The model under review builds one solid part; all positions refer to its coordinate system, in mm. Coordinates: 2 decimals unless noted, no trailing zeros. Write each loop counter-clockwise with the first axis right and the second up, starting at its lowest first coordinate (ties: lowest second). Pieces come first, ordered by that corner, then holes. Notation, with made-up numbers: (41, -37) - (88, -37) arc R10 cw to (88, -26) - close; hole circle Ø6 at (56, 26.25). An arc over 180 degrees is marked (long way). Put each result on its own line as item: value. Start each with the question number.
Item 1: Consider section B-B on y = 0.3. Give the boundary of the cut face in (x, z), then the cut area to 3 significant figures.
Item 2: Consider section A-A on z = 0. Give the boundary of the cut face in (x, y).
Item 3: To check wall thickness, follow L1, parallel to X at y = 1, z = 0; L2, parallel to Z at x = -6.25, y = 0.45; L3, parallel to X at y = 0.4, z = 4.5. State the ranges of each line that lie inside material, in increasing order. Write a range as [from, to].
Item 4: Consider section D-D on x = 0. Give the boundary of the cut face in (y, z), then the cut area to 3 significant figures.
Item 5: Consider section C-C on z = 3. Give the boundary of the cut face in (x, y), then the cut area to 3 significant figures.
```python
from build123d import *

# Parameters (mm, degrees)
EXTRUDE1_DEPTH = 1.2


with BuildPart() as part:
    # Sketch1 → Extrude1 (new body)
    with BuildSketch(Plane(origin=(0, 0, 0), x_dir=(1, 0, 0), z_dir=(0, 1, 0))):
        with BuildLine():
            Line((2.113091309, 4.531538935), (2.371939111, 5.086639839))
            ThreePointArc((2.371939111, 5.086639839), (3.208308367, 5.77268928), (4.266742072, 5.549316362))
            ThreePointArc((4.266742072, 5.549316362), (5.73406431, 4.015035054), (6.673963371, 2.111448062))
            ThreePointArc((6.673963371, 2.111448062), (6.515398476, 1.030863961), (5.568082875, 0.487358691))
            Line((5.568082875, 0.487358691), (4.979992479, 0.446849981))
            ThreePointArc((4.979992479, 0.446849981), (4.742221478, -1.58471936), (3.710828514, -3.351082175))
            Line((3.710828514, -3.351082175), (4.262184676, -6.810891939))
            ThreePointArc((4.262184676, -6.810891939), (5.05662557, -7.784180304), (6.29553407, -7.575536336))
            ThreePointArc((6.29553407, -7.575536336), (0, 9.85), (-6.29553407, -7.575536336))
            ThreePointArc((-6.29553407, -7.575536336), (-5.05662557, -7.784180304), (-4.262184676, -6.810891939))
            Line((-4.262184676, -6.810891939), (-3.710828514, -3.351082175))
            ThreePointArc((-3.710828514, -3.351082175), (-4.742221478, -1.58471936), (-4.979992479, 0.446849981))
            Line((-4.979992479, 0.446849981), (-5.568082875, 0.487358691))
            ThreePointArc((-5.568082875, 0.487358691), (-6.515398476, 1.030863961), (-6.673963371, 2.111448062))
            ThreePointArc((-6.673963371, 2.111448062), (-5.73406431, 4.015035054), (-4.266742072, 5.549316362))
            ThreePointArc((-4.266742072, 5.549316362), (-3.208308367, 5.77268928), (-2.371939111, 5.086639839))
            Line((-2.371939111, 5.086639839), (-2.113091309, 4.531538935))
            ThreePointArc((-2.113091309, 4.531538935), (0, 5), (2.113091309, 4.531538935))
        make_face()
    extrude(amount=EXTRUDE1_DEPTH)


solid = part.part
```
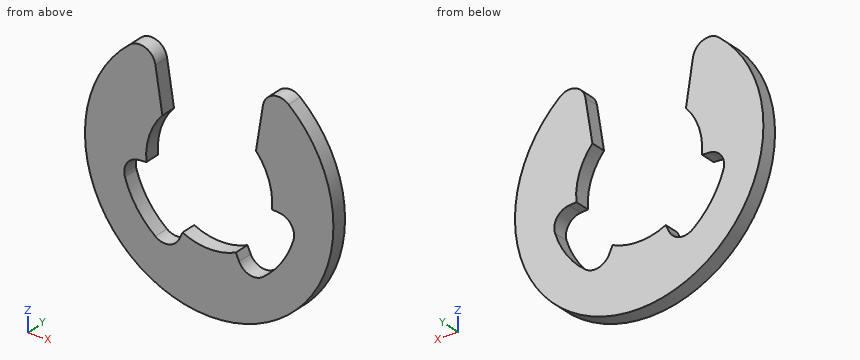
Report:
1. outline: (-6.67, -2.11) arc R1.25 cw to (-5.57, -0.49) - (-4.98, -0.45) arc R5 cw to (-3.71, 3.35) - (-4.26, 6.81) arc R1.25 ccw to (-6.3, 7.58) arc R9.85 ccw (long way) to (6.3, 7.58) arc R1.25 ccw to (4.26, 6.81) - (3.71, 3.35) arc R5 cw to (4.98, -0.45) - (5.57, -0.49) arc R1.25 cw to (6.67, -2.11) arc R7 cw to (4.27, -5.55) arc R1.25 cw to (2.37, -5.09) - (2.11, -4.53) arc R5 cw to (-2.11, -4.53) - (-2.37, -5.09) arc R1.25 cw to (-4.27, -5.55) arc R7 cw to start
1. area: 158 mm²
2. outline: (-9.85, 0) - (-5, 0) - (-5, 1.2) - (-9.85, 1.2) - close; (5, 0) - (9.85, 0) - (9.85, 1.2) - (5, 1.2) - close
3. L1: [-9.85, -5], [5, 9.85]
3. L2: [-7.61, -3.15], [-0.75, 7.61]
3. L3: [-8.76, -3.89], [3.89, 8.76]
4. outline: (0, -9.85) - (1.2, -9.85) - (1.2, -5) - (0, -5) - close
4. area: 5.82 mm²
5. outline: (-9.38, 0) - (-4, 0) - (-4, 1.2) - (-9.38, 1.2) - close; (4, 0) - (9.38, 0) - (9.38, 1.2) - (4, 1.2) - close
5. area: 12.9 mm²
